Source: CAD feature listing. Evaluate the final solid. Frame: model axes, mm. A direction names the side the tool comes from. Give positions to 0.01 mm unless a question says otherwise; leave off trailing zeros. Loops run counter-clockwise (first coordinate to the right, second up) from the corner with the lowest first, then second, coordinate; pieces in that order, holes last. Notation, with made-up numbers: (0, 42.5) -> (23, 42.5) arc R5 ccw to (23, 47.5) -> close; hole circle Ø2 at (8.5, -7.5). An arc over 180 degrees is marked (long way). Return JSON: item names as keys, results as strings. Group by question number.
Autodesk Inventor part; units mm, degrees
ref_plane "YZ Plane" through (0, 0, 0) normal (1, 0, 0) x (0, 1, 0)
ref_plane "XZ Plane" through (0, 0, 0) normal (0, 1, 0) x (-1, 0, 0)
ref_plane "XY Plane" through (0, 0, 0) normal (0, 0, 1) x (1, 0, 0)
sketch "Sketch1" plane through (0, 0, 0) normal (1, 0, 0) x (0, 1, 0)
  line L0 (292.1, 38.1) -> (-292.1, 38.1)
  line L1 (-292.1, 38.1) -> (-292.1, -38.1)
  line L2 (-292.1, -38.1) -> (292.1, -38.1)
  line L3 (292.1, -38.1) -> (292.1, 38.1)
  line L4 (-408.94, 0) -> (408.94, 0)
  line L5 (0, -53.34) -> (0, 53.34)
  point P0 (0, 0)
  dimension "d0" = 76.2
  dimension "d1" = 584.2
extrude "Plate1" add sketch "Sketch1" along normal blind 3.048
sketch "Sketch2" plane through (1.2881, 292.1, -35.3376) normal (-0.4226183, 0, -0.9063078) x (0, -1, 0)
  line L0 (584.2, 0) -> (0, 0)
  line L1 (0, 0) -> (0, -165.1)
  line L2 (0, -165.1) -> (584.2, -165.1)
  line L3 (584.2, -165.1) -> (584.2, 0)
edge flange "Flange1" height 165.1 angle 65 thickness 3.048 bend radius 3.048 thickness toward (-0.4226183, 0, -0.9063078) relief tear relief width 3.048 relief depth 1.524 corner gap 3.048 corner form 0 edges at (3.048, 0, -38.1) (3.048, 0, 38.1) wall of the first edge with corners at (1.2881, -292.1, -35.3376) (1.2881, 292.1, -35.3376) (150.9196, 292.1, -105.1118) (150.9196, -292.1, -105.1118)
bend "Bend1"
corner "Corner1"
sketch "Sketch3" plane through (147.8716, 292.1, 105.1118) normal (1, 0, 0) x (0, 1, 0)
  line L0 (-584.2, 0) -> (0, 0)
  line L1 (0, 0) -> (0, 25.4)
  line L2 (0, 25.4) -> (-584.2, 25.4)
  line L3 (-584.2, 25.4) -> (-584.2, 0)
edge flange "Flange2" height 25.4 angle 65 thickness 3.048 bend radius 3.048 thickness toward (1, 0, 0) relief tear relief width 3.048 relief depth 1.524 corner gap 3.048 corner form 0 edges at (149.6314, 0, 107.8743) (149.6314, 0, -107.8743) wall of the first edge with corners at (147.8716, -292.1, 105.1118) (147.8716, 292.1, 105.1118) (147.8716, 292.1, 130.5118) (147.8716, -292.1, 130.5118)
bend "Bend2"
corner "Corner2"
equation "\"d3\" = BendReliefWidth"
equation "\"d4\" = BendReliefDepth"
equation "\"d5\" = MinimumRemnant"
equation "\"d6\" = BendRadius"
equation "\"d9\" = BendRadius"
equation "\"d10\" = CornerReliefSize"
equation "\"d11\" = GapSize"
equation "\"d12\" = JacobiRadiusSize"
equation "\"d13\" = BendReliefWidth"
equation "\"d14\" = BendReliefDepth"
equation "\"d15\" = MinimumRemnant"
equation "\"d16\" = BendRadius"
equation "\"d19\" = BendRadius"
equation "\"d20\" = CornerReliefSize"
equation "\"d21\" = GapSize"
equation "\"d22\" = JacobiRadiusSize"
equation "\"BendRadius\" = Thickness"
equation "\"BendReliefWidth\" = Thickness"
equation "\"BendReliefDepth\" = 0.5 * Thickness"
equation "\"CornerReliefSize\" = 4 * Thickness"
equation "\"MinimumRemnant\" = 2 * Thickness"
equation "\"TransitionRadius\" = BendRadius"
equation "\"JacobiRadiusSize\" = BendRadius"
equation "\"GapSize\" = Thickness"
equation "\"d2\" = BendRadius"
properties part number "Bread Pan"
1) Mould query, pull axis Z, two halves, no side actions, for faces 1 (the face through (75.11, -4.09, 69.76)), 2 (the face through (3.048, -4, 0)), 3 (the face through (75.81, 4.09, -73.45)), 4 (the face through (150.92, 4, 120)). Classes: released by +Z, released by -Z, zero draft, split by the parting line, or undercut.
2) Reachability of faces 5 (the face through (66.1, 292.1, 68.7)), 6 (the face through (75.11, 4.09, -69.76)), 7 (the face through (66.1, -292.1, 68.7)), 8 (the face through (147.872, -4, -120)), 9 (the face through (147.872, 4, 120)) from +Z, -Z, +X, -X, +Y, -Y: full face, straight path, thin tool, end or side. Return the list, or none.
3) Material intervals for line 1 (X direction, y = 240, z = -19); line 2 (Z direction, x = 10.5, y = 144); line 3 (Z direction, x = 83, y = 161), sorted ascending.
4) Cut plane D-D on z = -73. Return loops of the section in (x, y).
5) Cut plane C-C on z = 27. Return loops of the section in (x, y).
6) Contact query for flat-ended pins moving along their axis: P1, Ø5, axis at y = 143.5, z = 38, coming from the +X side; P2, Ø3, axis at x = 85, y = 169, coming from the -Z side; P3, Ø12, axis at x = 109, y = 126.5, coming from the +Z side. Output: stop coordinate, or through.
7) Cut plane A-A on x = 111. Return loops of the section in (y, z).
8) Cut plane B-B on y = 88. Return loops of the section in (x, z), then the cut area to 3 significant figures.
Calculated:
{
 "1": {"face 1": "undercut", "face 2": "undercut", "face 3": "released by -Z", "face 4": "zero draft"},
 "2": {"face 5": "+Z, -Z, +X, -X, +Y", "face 6": "+X, +Y, -Y", "face 7": "+Z, -Z, +X, -X, -Y", "face 8": "-Z, -X, +Y, -Y", "face 9": "+Z, -X, +Y, -Y"},
 "3": {"line 1": "0 to 3.05", "line 2": "-43 to -39.63, 39.63 to 43", "line 3": "-76.8 to -73.44, 73.44 to 76.8"},
 "4": {"outline": "(74.84, -292.1) -> (82.06, -292.1) -> (82.06, 292.1) -> (74.84, 292.1) -> close"},
 "5": {"outline": "(0, -292.1) -> (3.05, -292.1) -> (3.05, 292.1) -> (0, 292.1) -> close"},
 "6": {"P1": "x = 12.36", "P2": "z = -78.44", "P3": "z = 91.73"},
 "7": {"outline": "(-292.1, -89.86) -> (292.1, -89.86) -> (292.1, -86.5) -> (-292.1, -86.5) -> close; (-292.1, 86.5) -> (292.1, 86.5) -> (292.1, 89.86) -> (-292.1, 89.86) -> close"},
 "8": {"outline": "(0, -34.22) arc R6.1 ccw to (3.52, -39.74) -> (146.11, -106.23) arc R3.05 cw to (147.87, -109) -> (147.87, -130.51) -> (150.92, -130.51) -> (150.92, -109) arc R6.1 ccw to (147.4, -103.47) -> (4.81, -36.98) arc R3.05 cw to (3.05, -34.22) -> (3.05, 34.22) arc R3.05 cw to (4.81, 36.98) -> (147.4, 103.47) arc R6.1 ccw to (150.92, 109) -> (150.92, 130.51) -> (147.87, 130.51) -> (147.87, 109) arc R3.05 cw to (146.11, 106.23) -> (3.52, 39.74) arc R6.1 ccw to (0, 34.22) -> close", "area": "1,360 mm2"}
}
